```python
from build123d import *

# Parameters (mm, degrees)
CYLINDER_R          = 12.7
CYLINDER_DEPTH      = 476.25
CYLINDER_ROLL_ANGLE = 90
THICKNESS001_T      = 6.35


with BuildPart() as part:
    # Cylinder → Cylinder (new body)
    with BuildSketch(Plane.XY):
        Circle(CYLINDER_R)
    extrude(amount=CYLINDER_DEPTH)


with BuildPart() as part_1:
    # Cylinder roll: moved
    add(part.part.rotate(Axis((0, 0, 0), (1, 0, 0)), CYLINDER_ROLL_ANGLE))


with BuildPart() as part_2:
    # Cylinder placement: moved
    add(part_1.part)

    # Thickness001
    thickness001_openings = [part_2.faces().sort_by_distance(p)[0] for p in [
        (0, 0, 0),
        (0, -476.25, 0),
    ]]
    offset(amount=THICKNESS001_T, openings=thickness001_openings)


solid = part_2.part
```
Read the model definition and answer for the solid it produces. Units are mm, in the model's axes. Give positions to 0.01 mm unless a question says otherwise; leave off trailing zeros. Loops run counter-clockwise (first coordinate to the right, second up) from the corner with the lowest first, then second, coordinate; pieces in that order, holes last.
Item 1: Each of these flat-tipped pins is pushed along its axis until it touches: pin 1 Ø1 at (x, y) = (7.5, -225) entering from -Z; pin 2 Ø10 at (y, z) = (-266.5, -13.5) entering from +X; pin 3 Ø2 at (x, y) = (-6, -408.5) entering from +Z; pin 4 Ø2 at (x, z) = (3, 10.5) entering from -Y. Where does it stop, or does it pass through?
Item 2: The part is cut by section A-A (z = 0). Write down the section's boundary in (x, y), and give its area (3 significant figures).
Item 3: Find the intervals of material crossed by line 1 along Z through (x, y) = (0, -150); line 2 along X through (y, z) = (-58, 1.5); line 3 along X through (y, z) = (-152.5, -6), in increasing order.
Item 4: The part is cut by section B-B (x = 0). Write down the section's boundary in (y, z).
Item 5: The part is cut by section C-C (y = -337.5). Write down the section's boundary in (x, z).
Item 6: The mould has two halves that part along X. Classify faces 1 (the cylindrical face through (-2.48, -234.791, 18.888)), 2 (the flat face through (12.4, 0, -4)), 3 (the cylindrical face through (12.114, -234.791, 3.815)): released by +X, released by -X, zero draft, split by the parting line, or undercut.
Taken from the geometry:
1. pin 1: stops at z = -17.72
1. pin 2: stops at x = 17.05
1. pin 3: stops at z = 18.38
1. pin 4: passes through
2. outline: (-19.05, -476.25) - (-12.7, -476.25) - (-12.7, 0) - (-19.05, 0) - close; (12.7, -476.25) - (19.05, -476.25) - (19.05, 0) - (12.7, 0) - close
2. area: 6,050 mm2
3. line 1: z = -19.05 to -12.7, 12.7 to 19.05
3. line 2: x = -18.99 to -12.61, 12.61 to 18.99
3. line 3: x = -18.08 to -11.19, 11.19 to 18.08
4. outline: (-476.25, -19.05) - (0, -19.05) - (0, -12.7) - (-476.25, -12.7) - close; (-476.25, 12.7) - (0, 12.7) - (0, 19.05) - (-476.25, 19.05) - close
5. outline: circle Ø38.1 at (0, 0); hole circle Ø25.4 at (0, 0)
6. face 1: split by the parting line
6. face 2: zero draft
6. face 3: undercut
